Geometry: final body of the model. Coordinates: model frame, mm. A direction names the side the tool comes from. Round coordinates to 2 decimals unless told otherwise and drop trailing zeros. Loops run counter-clockwise (first coordinate to the right, second up) from the corner with the lowest first, then second, coordinate; pieces in that order, holes last. Notation, with made-up numbers: (87, -18.75) - (109, -18.75) arc R28 cw to (109, 20.25) - close; hole circle Ø10 at (-11, -12). An arc over 180 degrees is marked (long way). Answer as CSV lines item,"result".
from build123d import *

# Parameters (mm, degrees)
SKETCH_1_R      = 10
SKETCH_1_R_2    = 5.5
EXTRUDE_1_DEPTH = 18.5
SKETCH_4_R      = 5
SKETCH_6_R      = 3
SKETCH_8_R      = 3
SKETCH_10_R     = 3


with BuildPart() as part:
    # Эскиз1 → Бобышка-Вытянуть1 (new body)
    with BuildSketch(Plane(origin=(0, 0, 0), x_dir=(0, 0, -1), z_dir=(1, 0, 0))):
        Circle(SKETCH_1_R)
        Circle(SKETCH_1_R_2, mode=Mode.SUBTRACT)
    extrude(amount=EXTRUDE_1_DEPTH)

    # По траектории1: sweep along a curve in space
    with BuildLine() as sweep_1_path:
        Line((9, -16.912295169, 41.627726505), (9, -31.601007166, 81.984631039))
        ThreePointArc((9, -14.5, 27.946920772), (9, -15.10768988, 34.892847878), (9, -16.912295169, 41.627726505))
        Line((9, -14.5, 27.946920772), (9, -14.5, -34.021959946))
        ThreePointArc((9, -14.5, -34.021959946), (8.560634534, -14.5, -39.934336391), (7.252190239, -14.5, -45.716828135))
        Line((7.252190239, -14.5, -45.716828135), (-10.881275921, -14.5, -105.028723405))
    # Эскиз4 → По траектории1 (sweep)
    with BuildSketch(Plane.XY):
        with Locations((9, -14.5)):
            Circle(SKETCH_4_R)
    sweep(path=sweep_1_path.line)

    # По траектории2: sweep along a path in Эскиз5
    with BuildLine(Plane(origin=(0, -9.5, 0), x_dir=(1, 0, 0), z_dir=(0, 1, 0))) as sweep_2_path:
        ThreePointArc((9.327108594, 149.328764781), (-10.881275921, 105.028723405), (-52.407054726, 130.45473696))
    # Эскиз6 → По траектории2 (sweep)
    with BuildSketch(Plane(origin=(-52.407054726, -9.5, -130.45473696), x_dir=(-0.984679674516163, 0, 0.17437298699839734), z_dir=(-0.17437298699839734, 0, -0.984679674516163))):
        Circle(SKETCH_6_R)
    sweep(path=sweep_2_path.line)

    # По траектории4: sweep along a path in Эскиз7
    with BuildLine(Plane(origin=(0, -9.5, 0), x_dir=(1, 0, 0), z_dir=(0, 1, 0))) as sweep_4_path:
        Line((-6.948042364, 144.352951788), (12.068642346, 150.546957166))
    # Эскиз8 → По траектории4 (sweep)
    with BuildSketch(Plane(origin=(-6.948042364, -9.5, -144.352951788), x_dir=(-0.2923717047227386, 0, -0.9563047559630349), z_dir=(0.9563047559630349, 0, -0.2923717047227386))):
        Circle(SKETCH_8_R)
    sweep(path=sweep_4_path.line)

    # По траектории5: sweep along a path in Эскиз9
    with BuildLine(Plane(origin=(0, -9.5, 0), x_dir=(1, 0, 0), z_dir=(0, 1, 0))) as sweep_5_path:
        Line((-36.131903768, 135.430549953), (-55.36109375, 129.931617999))
    # Эскиз10 → По траектории5 (sweep)
    with BuildSketch(Plane(origin=(-36.131903768, -9.5, -135.430549953), x_dir=(-0.2923717047227386, 0, -0.9563047559630349), z_dir=(0.9563047559630349, 0, -0.2923717047227386))):
        Circle(SKETCH_10_R)
    sweep(path=sweep_5_path.line)


solid = part.part
(1) Section A-A (y = 0). Output: boundary loops of the cut face in (x, z).
Findings below:
outline,"(0, -10) - (18.5, -10) - (18.5, -5.5) - (0, -5.5) - close; (0, 5.5) - (18.5, 5.5) - (18.5, 10) - (0, 10) - close"
(2) Material intervals for line 1 along Y through (x, z) = (5, 0); line 2 along Z through (x, y) = (2.5, -1); line 3 along Z through (x, y) = (3, -8), sorted ascending.
Findings below:
line 1,"-17.5 to -11.5, -10 to -5.5, 5.5 to 10"
line 2,"-9.95 to -5.41, 5.41 to 9.95"
line 3,"-150.33 to -144.86, -117.47 to -109.93, -6 to 6"
(3) Draft query along Z for faces 5 (the face through (9.12, -5.37, 1.19)), 6 (the face through (-36, -10, -135)), 7 (the face through (18.5, -4, -4)). Return one class per face: pulls with the +Z half, pulls with the -Z half, needs draft (parallel to the pull), parting line crosses it, or undercut.
Findings below:
face 5,"undercut"
face 6,"pulls with the -Z half"
face 7,"needs draft"
(4) Section C-C (x = -3.5). Give the number of separate pieces and of enclosed holes in the cut face, and give its area (3 significant figures).
Findings below:
separate pieces,"3"
enclosed holes,"0"
area,"332 mm2"
(5) Pin query (flat end, axial travel): P1, Ø16, axis at y = 2, z = 2.5, coming from the -X side; P2, Ø5, axis at x = 8, z = -108, coming from the +Y side; P3, Ø12.5, axis at y = 0, z = 0, coming from the +X side; P4, Ø5, axis at y = -17, z = -76, coming from the -X side. Return the tip coordinate at first contact, or that it passes through.
Findings below:
P1,"x = 0"
P2,"through"
P3,"x = 18.5"
P4,"x = -7.74"
(6) Access query for faces 1 (the face through (-55.406, -9.542, -130.079)), 2 (the face through (12.023, -9.542, -150.695)), 3 (the face through (11.307, -18.936, -2.604)), 4 (the face through (0, -4, -4)). Directions: +Z, -Z, +X, -X, +Y, -Y. A direction counts if a zero-diameter tool reaches every point of the face in a straight line with its end or side. Return the directions, or none.
Findings below:
face 1,"+Z, -X"
face 2,"-Z, +X"
face 3,"none"
face 4,"+Z, -X, +Y, -Y"
(7) Section B-B (z = 0). Output: boundary loops of the cut face in (x, y), and give its area (3 significant figures).
Findings below:
outline,"(0, -10) - (6.82, -10) arc R5 ccw (long way) to (11.18, -10) - (18.5, -10) - (18.5, -5.5) - (0, -5.5) - close; (0, 5.5) - (18.5, 5.5) - (18.5, 10) - (0, 10) - close"
area,"244 mm2"
